from build123d import *

# Parameters (mm, degrees)
F2_SIZE  = 3
F3_W     = 30
F3_H     = 8.326223
F3_H_2   = 2
F4_DEPTH = 15
F6_DEPTH = 15


with BuildPart() as f1:
    # F0 (on Front) → F1 (revolve)
    with BuildSketch(Plane.XZ):
        Polygon((-40, 8), (-40, 0), (10, 0), (10, 14), (0, 14), (0, 8), align=None)
    revolve(axis=Axis((-23.084291, 0, 0), (-1, 0, 0)))

    # F2
    f2_edges = [f1.edges().sort_by_distance(p)[0] for p in [
        (10, 0, -14),
    ]]
    chamfer(f2_edges, length=F2_SIZE)

    # F3 (on Front) → F4 (cut, symmetric)
    with BuildSketch(Plane.XZ):
        with Locations((-5, 12.163677)):
            Rectangle(F3_W, F3_H)
        with Locations((-5, 7.000566)):
            Rectangle(F3_W, F3_H_2)
    extrude(amount=F4_DEPTH, both=True, mode=Mode.SUBTRACT)

    # F5 (on Front) → F6 (cut, symmetric)
    with BuildSketch(Plane.XZ):
        Polygon((-24, 8), (-40, 8), (-40, -8), align=None)
    extrude(amount=F6_DEPTH, both=True, mode=Mode.SUBTRACT)


solid = f1.part
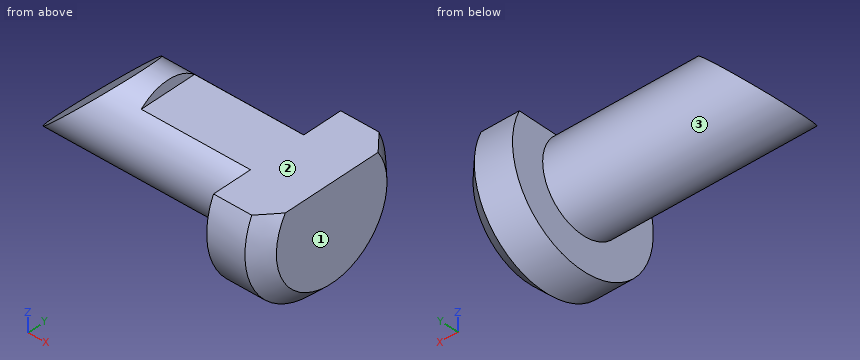
Geometry: final body of the model. Coordinates: model frame, mm. Face numbers are marked on the shaded views. A direction names the side the tool comes from. Round coordinates to 2 decimals unless told otherwise and drop trailing zeros. Order: outer loops, then holes, each group sorted by start corner. A loop starts at its lowest first (then second) coordinate and runs counter-clockwise, first axis right, second up. Notation, with made-up numbers: (23, 39) -> (67, 39) arc R14 ccw to (67, 66) -> close; hole circle Ø7 at (-30.5, 30.5). An arc over 180 degrees is marked (long way). Put each result on its own line as item: value. Start each with the question number.
Q1. First-contact query: pin 1 (2 mm diameter, centred on y = -1, z = 7.5, fed in from +X); pin 2 (6 mm diameter, centred on x = -12, y = 2, fed in from +Z); pin 3 (3 mm diameter, centred on x = 4.5, z = -5.5, fed in from -Y). Flat tips, straight axial feed; report the tip coordinate or a pass-through.
Q2. Reachability of the marked faces 1, 2 and 3 from +Z, -Z, +X, -X, +Y, -Y: full face, straight path, thin tool, end or side. Return the list, or none.
Q3. Line query: probe 1 along X at (y, z) = (-9.75, 1.75); probe 2 along Y at (x, z) = (-15, -6); probe 3 along Y at (x, z) = (2.5, 3). Output: solid intervals per line, ascending.
Q4. Section C-C on x = -8. Return the cut outline in (y, z).
Q5. Section B-B on x = 2. Return the cut outline in (y, z), and give its area (3 significant figures).
Q6. Section A-A on y = 0. Return the cut outline in (x, z).
Ans:
1. pin 1: stops at x = -20
1. pin 2: stops at z = 6
1. pin 3: stops at y = -13.42
2. face 1: +Z, -Z, +X, +Y, -Y
2. face 2: +Z, +X, +Y, -Y
2. face 3: -X
3. probe 1: x = 0 to 10
3. probe 2: y = -5.29 to 5.29
3. probe 3: y = -13.67 to 13.67
4. outline: (-5.29, 6) arc R8 ccw (long way) to (5.29, 6) -> close
5. outline: (-12.65, 6) arc R14 ccw (long way) to (12.65, 6) -> close
5. area: 471 mm2
6. outline: (-40, -8) -> (0, -8) -> (0, -14) -> (7, -14) -> (10, -11) -> (10, 6) -> (-20, 6) -> (-20, 8) -> (-24, 8) -> close
